Drawing for the job (mm, zero at the part's lowest x, y, z). Coordinates: 2 decimals unless noted, no trailing zeros. Write each loop counter-clockwise with the first axis right and the second up, starting at its lowest first coordinate (ties: lowest second). Pieces come first, ordered by that corner, then holes.
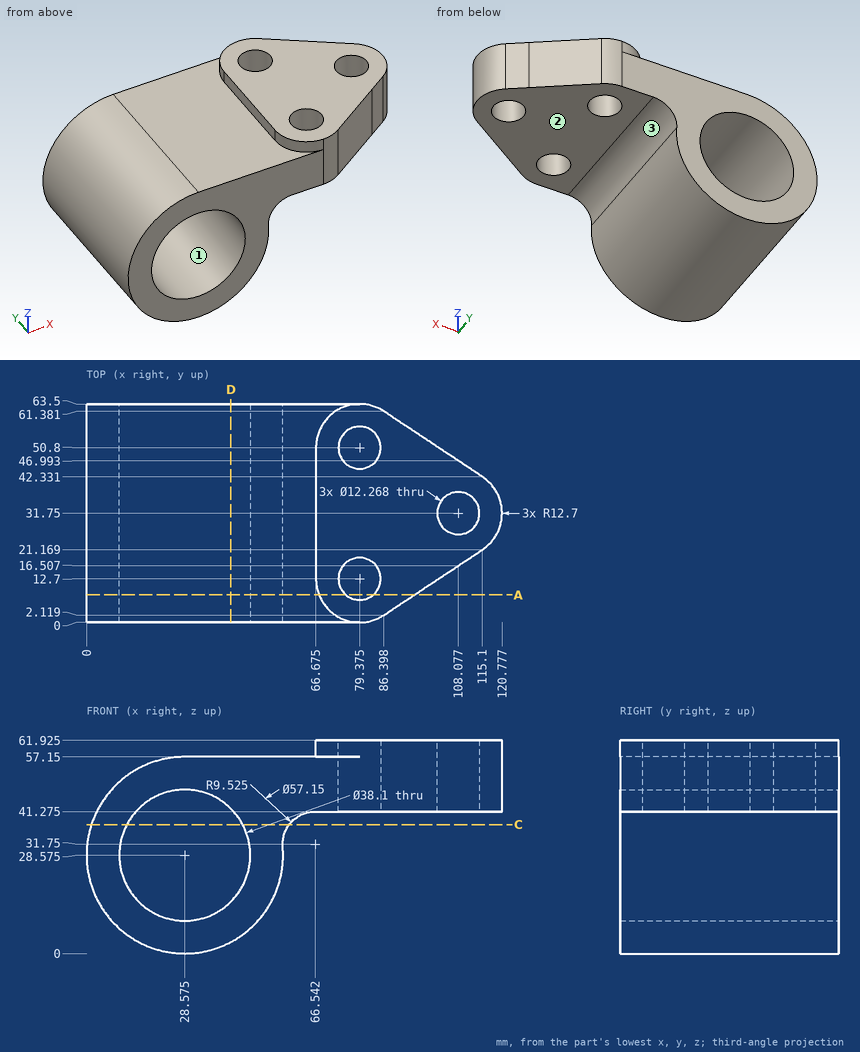
Item 1: Wall check: line 1 along Y through (x, z) = (80, 59.5) (1 decimal); line 2 along X through (y, z) = (14, 29.5) (1 decimal); line 3 along Z through (x, y) = (84.5, 32.5) (1 decimal). Give the ranges that are in metal, low to high.
Item 2: Flat gauge pins, fed straight in: pin 1 Ø8 at (y, z) = (44.5, 33) entering from +X (1 decimal); pin 2 Ø1 at (y, z) = (16, 31) entering from +X (1 decimal); pin 3 Ø7.5 at (x, y) = (108.077, 31.75) entering from +Z; pin 4 Ø4 at (y, z) = (27.5, 13) entering from -X. Where does each tip first touch, or does it go through?
Item 3: Saw through at C-C, the plane z = 37.5. Write the cut outline in (x, y) (1 decimal).
Item 4: Saw through at D-D, the plane x = 42. Write the cut outline in (y, z).
Item 5: Saw through at A-A, the plane y = 8. State how many separate pieces and enclosed holes the cut face has, and give its area (3 significant figures).
Item 6: Two-plate mould, pull along X, no slides. Class the marked faces 1, 2 and 3: +X half, -X half, draft (parallel to the pull), parting line (faces both ways), or undercut.
Working result:
1. line 1: y = 0 to 6.6, 18.8 to 44.7, 56.9 to 63.5
1. line 2: x = 0 to 9.5, 47.6 to 57.1
1. line 3: z = 41.3 to 61.9
2. pin 1: stops at x = 58.6
2. pin 2: stops at x = 57.1
2. pin 3: passes through
2. pin 4: stops at x = 3.43
3. outline: (1.4, 0) - (11.7, 0) - (11.7, 63.5) - (1.4, 63.5) - close; (45.4, 0) - (58.9, 0) - (58.9, 63.5) - (45.4, 63.5) - close
4. outline: (0, 3.35) - (63.5, 3.35) - (63.5, 15.06) - (0, 15.06) - close; (0, 42.09) - (63.5, 42.09) - (63.5, 57.15) - (0, 57.15) - close
5. separate pieces: 2
5. enclosed holes: 1
5. area: 2,190 mm2
6. face 1: undercut
6. face 2: draft
6. face 3: +X half
